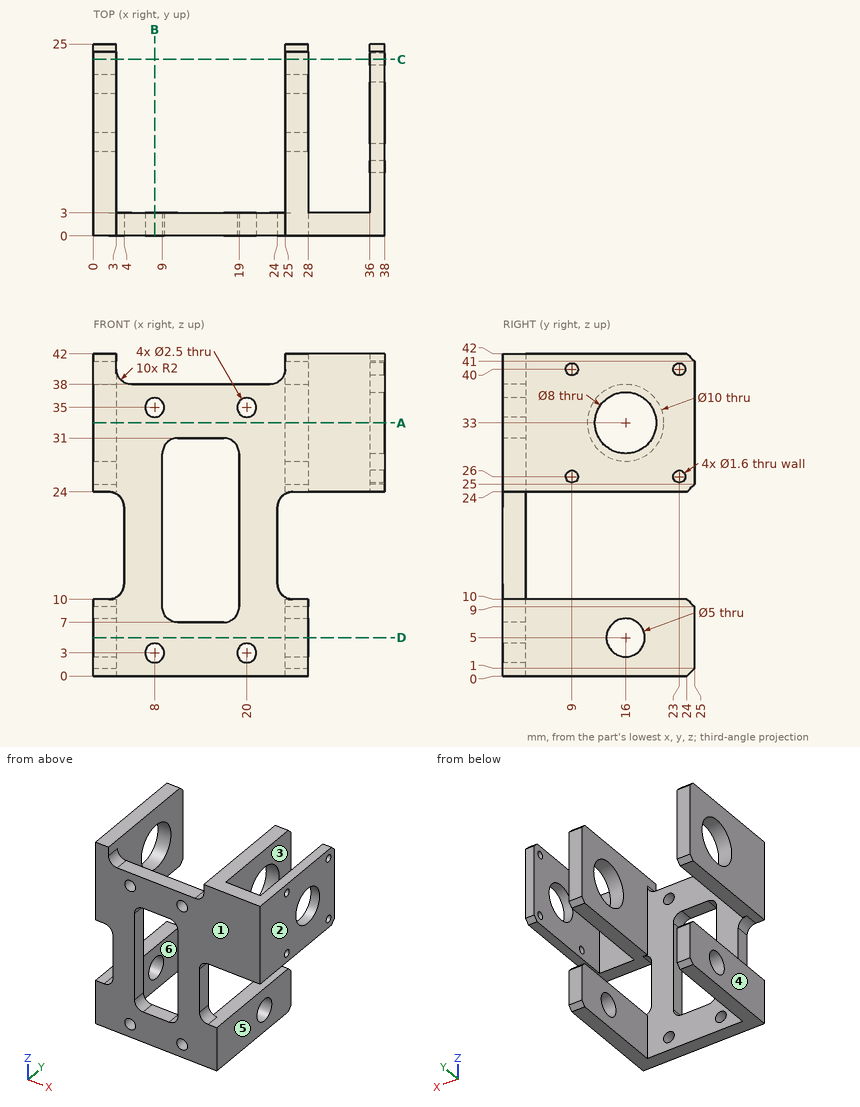
Drawing for the job (mm, zero at the part's lowest x, y, z). A direction names the side the tool comes from. Give positions to 0.01 mm unless a question says otherwise; leave off trailing zeros. Loops run counter-clockwise (first coordinate to the right, second up) from the corner with the lowest first, then second, coordinate; pieces in that order, holes last.
Item 1: Slice it at C-C (y = 23). Write the cut outline in (x, z).
Check values:
outline: (0, 0) - (3, 0) - (3, 10) - (0, 10) - close; (0, 24) - (3, 24) - (3, 42) - (0, 42) - close; (25, 0) - (28, 0) - (28, 10) - (25, 10) - close; (25, 24) - (28, 24) - (28, 42) - (25, 42) - close; (36, 24) - (38, 24) - (38, 25.2) - (36, 25.2) - close; (36, 26.8) - (38, 26.8) - (38, 39.2) - (36, 39.2) - close; (36, 40.8) - (38, 40.8) - (38, 42) - (36, 42) - close
Item 2: Which spindle directions (+Z, -Z, +X, -X, +Y, -Y) get a long thin tool onto all of the face, cutting with end or side? Do the marked faces 4, 5 and 6. Say none if no direction does.
Check values:
face 4: +Z, -Z, -X, +Y, -Y
face 5: -Z, +X, +Y, -Y
face 6: +Z, -Z, +Y
Item 3: Slice it at D-D (z = 5). Write the cut outline in (x, y), plus the area to 3 significant figures.
Check values:
outline: (0, 0) - (28, 0) - (28, 13.5) - (25, 13.5) - (25, 3) - (3, 3) - (3, 13.5) - (0, 13.5) - close; (0, 18.5) - (3, 18.5) - (3, 25) - (0, 25) - close; (25, 18.5) - (28, 18.5) - (28, 25) - (25, 25) - close
area: 186 mm2
Item 4: Drop flat-ended pins along their axis: P1, Ø6, axis at y = 22, z = 31.5, coming from the -X side; P2, Ø0.9, axis at y = 1.5, z = 17.5, coming from the -X side; P3, Ø1, axis at x = 20, z = 7, coming from the +Y side; P4, Ø1.5, axis at x = 13, y = 2, coming from the +Z side. Give the stop position or say it passes through.
Check values:
P1: stops at x = 0
P2: stops at x = 4
P3: stops at y = 3
P4: stops at z = 38
Item 5: Slice it at A-A (z = 33). Write the cut outline in (x, y).
Check values:
outline: (0, 0) - (38, 0) - (38, 12) - (36, 12) - (36, 3) - (28, 3) - (28, 11) - (25, 11) - (25, 3) - (3, 3) - (3, 11) - (0, 11) - close; (0, 21) - (3, 21) - (3, 25) - (0, 25) - close; (25, 21) - (28, 21) - (28, 25) - (25, 25) - close; (36, 20) - (38, 20) - (38, 25) - (36, 25) - close
Item 6: Slice it at B-B (x = 8). Write the cut outline in (y, z).
Check values:
outline: (0, 0) - (3, 0) - (3, 1.75) - (0, 1.75) - close; (0, 4.25) - (3, 4.25) - (3, 33.75) - (0, 33.75) - close; (0, 36.25) - (3, 36.25) - (3, 38) - (0, 38) - close
Item 7: Mould opens along X. For the marked faces 1, 2 and 3 say: +X half, -X half, draft (parallel to the pull), parting line (faces both ways), or undercut.
Check values:
face 1: draft
face 2: +X half
face 3: undercut
Item 8: Drill centre lines: line 1 along X through (y, z) = (9.5, 25); line 2 along Z through (x, y) = (36.65, 23); line 3 along Y through (x, z) = (37, 40). Where is each one in solid material? Low to high.
Check values:
line 1: x = 0 to 3, 25 to 28, 36 to 38
line 2: z = 24 to 25.2, 26.8 to 39.2, 40.8 to 42
line 3: y = 0 to 8.2, 9.8 to 22.2, 23.8 to 25
